Part model, mm, in its own coordinate system. Coordinates: 2 decimals unless noted, no trailing zeros. Write each loop counter-clockwise with the first axis right and the second up, starting at its lowest first coordinate (ties: lowest second). Pieces come first, ordered by that corner, then holes. Notation, with made-up numbers: M 43.5,19.5 L 63.5,19.5 A17 ccw 63.5,43.5 Z; hole C -37,-20.75 d2. An arc over 180 degrees is marked long. Use a Markdown table: item, result. Add a question column.
Q1. Slice it at A-A on x = 0. Write the cut outline in (y, z).
Q2. Slice it at C-C on z = 74. Count the separate pieces of the cut face and the enclosed holes in it, then the cut area to 3 significant figures.
Q3. Pin check, flat tips, straight feed: pin 1 Ø3 at (x, y) = (5, -1.5) entering from +Z; pin 2 Ø4 at (y, z) = (2.5, 104) entering from +X; pin 3 Ø1 at (x, y) = (7, 3) entering from +Z; pin 4 Ø3 at (x, z) = (0, 100.5) entering from +Y. Stop position of each tip, or through.
Q4. Wall check: L1, parallel to Y at x = 0, z = 130.5; L2, parallel to X at y = 8.25, z = 213; L3, parallel to X at y = -3.75, z = 29. Give the ranges that are in metal, low to high. Write a range as from..to.
Q5. Mould opens along Y. For faces 1 (the flat face through (0, 3.901, 123)), 2 (the flat face through (-0.1, 2.4, 250)), 3 (the cylindrical face through (2.003, -0.631, 123.25)), 4 (the flat face through (3.901, 0, 123)) say: released by +Y, released by -Y, zero draft, split by the parting line, or undercut.
Autodesk Inventor part; units mm, degrees
ref_plane "Start Plane" through (0, 0, 0) normal (0, 0, 1) x (1, 0, 0)
ref_plane "End Plane" through (0, 0, 20) normal (0, 0, 1) x (1, 0, 0)
ref_plane "YZ Plane" through (0, 0, 0) normal (1, 0, 0) x (0, 1, 0)
sketch "Sketch1" plane through (0, 0, 0) normal (0, 0, 1) x (1, 0, 0)
  line L0 (10, -4.5951) -> (10, -8.2)
  line L1 (-10, -8.2) -> (-10, -4.5951)
  line L2 (-10, 10) -> (10, -10) construction
  line L3 (10, 10) -> (-10, -10) construction
  circle A0 centre (0, 0) radius 2.1
  line L4 (-2.84, -3.9007) -> (2.84, -3.9007)
  line L5 (3.9007, -2.84) -> (3.9007, 2.84)
  line L6 (2.84, 3.9007) -> (-2.84, 3.9007)
  line L7 (-3.9007, 2.84) -> (-3.9007, -2.84)
  line L8 (-3.9007, -3.9007) -> (3.9007, 3.9007) construction
  line L9 (3.9007, -3.9007) -> (-3.9007, 3.9007) construction
  line L10 (-3.9007, -2.84) -> (-2.84, -3.9007) construction
  line L11 (-2.84, -3.9007) -> (-5.4993, -6.56)
  line L12 (-5.4993, -6.56) -> (-5.4993, -8.2)
  line L13 (-5.4993, -8.2) -> (-2.7951, -8.2)
  line L14 (-2.7951, -8.2) -> (-4.5951, -10)
  line L15 (0, 0) -> (0, -3.9007) construction
  line L16 (3.9007, -2.84) -> (2.84, -3.9007) construction
  line L17 (2.84, -3.9007) -> (5.4993, -6.56)
  line L18 (5.4993, -6.56) -> (5.4993, -8.2)
  line L19 (5.4993, -8.2) -> (2.7951, -8.2)
  line L20 (2.7951, -8.2) -> (4.5951, -10)
  line L21 (-2.84, -3.9007) -> (-3.9007, -2.84) construction
  line L22 (-3.9007, -2.84) -> (-6.56, -5.4993)
  line L23 (-6.56, -5.4993) -> (-8.2, -5.4993)
  line L24 (-8.2, -5.4993) -> (-8.2, -2.7951)
  line L25 (-8.2, -2.7951) -> (-10, -4.5951)
  line L26 (3.9007, -2.84) -> (6.56, -5.4993)
  line L27 (6.56, -5.4993) -> (8.2, -5.4993)
  line L28 (8.2, -5.4993) -> (8.2, -2.7951)
  line L29 (8.2, -2.7951) -> (10, -4.5951)
  arc A1 (-10, -8.2) -> (-8.2, -10) centre (-8.2, -8.2) ccw
  arc A2 (8.2, -10) -> (10, -8.2) centre (8.2, -8.2) ccw
  line L30 (-8.2, -6.56) -> (-7.7111, -6.56)
  line L31 (-6.6505, -8.2) -> (-8.2, -8.2)
  line L32 (-8.2, -8.2) -> (-8.2, -6.56)
  line L33 (-6.6505, -7.6207) -> (-7.7111, -6.56)
  line L34 (-6.6505, -7.6207) -> (-6.6505, -8.2)
  line L35 (8.2, -6.56) -> (7.7111, -6.56)
  line L36 (6.6505, -8.2) -> (8.2, -8.2)
  line L37 (8.2, -8.2) -> (8.2, -6.56)
  line L38 (6.6505, -7.6207) -> (7.7111, -6.56)
  line L39 (6.6505, -7.6207) -> (6.6505, -8.2)
  line L40 (8.2, -10) -> (4.5951, -10)
  line L41 (-4.5951, -10) -> (-8.2, -10)
  line L42 (-3.9007, 0) -> (3.9007, 0) construction
  line L43 (10, 4.5951) -> (10, 8.2)
  line L44 (-10, 8.2) -> (-10, 4.5951)
  line L45 (-2.84, 3.9007) -> (2.84, 3.9007)
  line L46 (-3.9007, 2.84) -> (-2.84, 3.9007) construction
  line L47 (-2.84, 3.9007) -> (-5.4993, 6.56)
  line L48 (-5.4993, 6.56) -> (-5.4993, 8.2)
  line L49 (-5.4993, 8.2) -> (-2.7951, 8.2)
  line L50 (-2.7951, 8.2) -> (-4.5951, 10)
  line L51 (2.84, 3.9007) -> (5.4993, 6.56)
  line L52 (5.4993, 6.56) -> (5.4993, 8.2)
  line L53 (5.4993, 8.2) -> (2.7951, 8.2)
  line L54 (2.7951, 8.2) -> (4.5951, 10)
  line L55 (3.9007, 2.84) -> (2.84, 3.9007) construction
  line L56 (-8.2, 2.7951) -> (-10, 4.5951)
  line L57 (-2.84, 3.9007) -> (-3.9007, 2.84) construction
  line L58 (-3.9007, 2.84) -> (-6.56, 5.4993)
  line L59 (-6.56, 5.4993) -> (-8.2, 5.4993)
  line L60 (-8.2, 5.4993) -> (-8.2, 2.7951)
  line L61 (3.9007, 2.84) -> (6.56, 5.4993)
  line L62 (6.56, 5.4993) -> (8.2, 5.4993)
  line L63 (8.2, 5.4993) -> (8.2, 2.7951)
  line L64 (8.2, 2.7951) -> (10, 4.5951)
  arc A3 (-8.2, 10) -> (-10, 8.2) centre (-8.2, 8.2) ccw
  arc A4 (10, 8.2) -> (8.2, 10) centre (8.2, 8.2) ccw
  line L65 (-8.2, 6.56) -> (-7.7111, 6.56)
  line L66 (-6.6505, 8.2) -> (-8.2, 8.2)
  line L67 (-8.2, 8.2) -> (-8.2, 6.56)
  line L68 (-6.6505, 7.6207) -> (-7.7111, 6.56)
  line L69 (-6.6505, 7.6207) -> (-6.6505, 8.2)
  line L70 (8.2, 6.56) -> (7.7111, 6.56)
  line L71 (6.6505, 7.6207) -> (7.7111, 6.56)
  line L72 (8.2, 8.2) -> (8.2, 6.56)
  line L73 (6.6505, 7.6207) -> (6.6505, 8.2)
  line L74 (6.6505, 8.2) -> (8.2, 8.2)
  line L75 (8.2, 10) -> (4.5951, 10)
  line L76 (-4.5951, 10) -> (-8.2, 10)
  line L77 (-8.2, 10) -> (-4.5951, 10)
  line L78 (4.5951, 10) -> (8.2, 10)
  point P0 (8.2, -8.2)
  point P1 (0, 3.9007)
  point P2 (8.2, 8.2)
  point P3 (0, 2.1)
  point P4 (1.4849, 1.4849)
  point P5 (0, 2.1)
  point P6 (0, 10)
  dimension "Width" = 20
  dimension "Height" = 20
  dimension "d2" = 4.2
  dimension "d3" = 1.5
  dimension "d4" = 1.64
  dimension "d6" = 5.68
  dimension "d7" = 1.8
  dimension "d9" = 1.5
ref_plane "Start Plane" through (0, 0, 0) normal (0, 0, 1) x (1, 0, 0)
ref_plane "End Plane" through (0, 0, 20) normal (0, 0, 1) x (1, 0, 0)
sketch "Sketch4" plane through (0, 0, 0) normal (0, 0, 1) x (1, 0, 0)
  line L0 (0, 0) -> (10, 0)
ref_plane "Work Plane4" through (0, 0, 0) normal (0, -1, 0) x (1, 0, 0)
sketch "Sketch5" plane through (0, 0, 0) normal (0, -1, 0) x (1, 0, 0)
  line L0 (-2, 0) -> (12, 0) construction
  line L1 (-2, 20) -> (12, 20) construction
  dimension "d17" = 20
extrude "Extrusion3" add sketch "Sketch1" along normal blind 250
equation "\"G_OFFSET_START\" = 0"
equation "\"G_OFFSET_END\" = 0"
equation "\"G_L\" = d17"
properties part number "V-slot 20 mm x 20 mm" material "Aluminum 6061"
Recorded:
| question | item | result |
|---|---|---|
| 1 | outline | M -3.9,0 L -2.1,0 L -2.1,250 L -3.9,250 Z; M 2.1,0 L 3.9,0 L 3.9,250 L 2.1,250 Z |
| 2 | separate pieces | 1 |
| 2 | enclosed holes | 5 |
| 2 | area | 161 mm² |
| 3 | pin 1 | z = 250 |
| 3 | pin 2 | x = 9.9 |
| 3 | pin 3 | through |
| 3 | pin 4 | y = 3.9 |
| 4 | L1 | -3.9..-2.1, 2.1..3.9 |
| 4 | L2 | -10..-2.85, 2.85..10 |
| 4 | L3 | -9.15..-8.2, -4.81..4.81, 8.2..9.15 |
| 5 | face 1 | released by +Y |
| 5 | face 2 | zero draft |
| 5 | face 3 | undercut |
| 5 | face 4 | undercut |
